Autodesk Inventor part; units mm, degrees
ref_plane "YZ Plane" through (0, 0, 0) normal (1, 0, 0) x (0, 1, 0)
ref_plane "XZ Plane" through (0, 0, 0) normal (0, 1, 0) x (-1, 0, 0)
ref_plane "XY Plane" through (0, 0, 0) normal (0, 0, 1) x (1, 0, 0)
sketch "Sketch1" plane through (0, 0, 0) normal (0, 1, 0) x (-1, 0, 0)
  line L0 (10, 67.88) -> (-10, 67.88)
  line L1 (-10, 67.88) -> (-10, -10)
  line L2 (-10, -10) -> (10, -10)
  line L3 (10, -10) -> (10, 67.88)
  point P0 (0, 0)
  dimension "d0" = 20
  dimension "d1" = 77.88
extrude "Extrusion1" add sketch "Sketch1" along normal blind 2
sketch "Sketch2" plane through (0, 2, 0) normal (0, 1, 0) x (1, 0, 0)
  line L0 (-10, -67.88) -> (10, -67.88)
  line L1 (0, -67.88) -> (-6.35, -67.88)
  line L2 (-6.35, -56.98) -> (6.35, -56.98)
  line L3 (6.35, -67.88) -> (0, -67.88)
  line L4 (10, 10) -> (-10, 10)
  line L5 (-6.35, -0.9) -> (6.35, -0.9)
  line L6 (-6.35, 10) -> (6.35, 10)
  line L7 (-6.35, -67.88) -> (-10, -67.88)
  line L8 (-10, 10) -> (-10, -67.88)
  line L9 (-10, -56.98) -> (-6.35, -56.98)
  line L10 (6.35, -67.88) -> (10, -67.88)
  line L11 (10, -67.88) -> (10, 10)
  line L12 (10, -56.98) -> (6.35, -56.98)
  line L13 (6.35, -0.9) -> (10, -0.9)
  line L14 (10, 10) -> (6.35, 10)
  line L15 (10, -0.9) -> (10, 10)
  line L16 (10, -67.88) -> (10, -56.98)
  line L17 (-10, -67.88) -> (-10, -56.98)
  line L18 (-6.35, -0.9) -> (-10, -0.9)
  line L19 (-10, -0.9) -> (-10, 10)
  line L20 (-10, 10) -> (-6.35, 10)
  point P0 (0, 0)
  dimension "d4" = 6.35
  dimension "d5" = 10.9
  dimension "d6" = 12.7
  dimension "d7" = 10.9
extrude "Extrusion2" add sketch "Sketch2" along normal blind 43.3354 contours L8 L9 L2 L12 L11 L0 | L8 L4 L11 L13 L5 L18
sketch "Sketch9" plane through (-10, 0, 67.88) normal (0, 0, 1) x (1, 0, 0)
  arc A0 (15.084, 37.3223) -> (4.684, 37.3223) centre (9.884, 37.3223) ccw
  line L0 (15.084, 30.9243) -> (15.084, 37.3223)
  line L1 (4.684, 36.1247) -> (4.684, 37.3223)
  arc A1 (15.084, 37.3223) -> (4.684, 37.3223) centre (9.884, 37.3223) ccw
  line L2 (4.684, 37.3223) -> (4.684, 30.9247)
  line L3 (9.8815, 15.3222) -> (-0.0013, 15.3222)
  line L4 (-0.0013, 25.726) -> (-0.0013, 15.3222)
  line L5 (4.684, 30.9247) -> (4.684, 25.726)
  line L6 (15.084, 30.9243) -> (15.0845, 20.5254)
  arc A2 (15.084, 30.9243) -> (15.084, 30.9251) centre (9.884, 30.9244) ccw
  line L7 (4.684, 25.726) -> (-0.0013, 25.726)
  arc A3 (9.8815, 15.3222) -> (15.0845, 20.5254) centre (9.8815, 20.5252) ccw
  line L8 (0, 0) -> (20, 0)
  line L9 (0, 45.3354) -> (20, 45.3354)
  point P0 (10, 0)
  point P1 (2.3413, 25.726)
  point P2 (15.084, 30.9247)
  point P3 (9.884, 42.5223)
  point P4 (-0.0013, 20.5241)
  point P5 (10, 45.3354)
  dimension "d76" = 15.3222
  dimension "d77" = 10.4039
  dimension "d78" = 10.4
  dimension "d79" = 27.2001
  dimension "d80" = 15.0858
  dimension "d81" = 8.0131
fillet "Fillet4" radius 10 4 edges at (10, 45.3354, 62.43) (-10, 45.3354, 62.43) (-10, 45.3354, -4.55) (10, 45.3354, -4.55)
sketch "Sketch10" plane through (0, 2, 0) normal (0, 1, 0) x (1, 0, 0)
  line L0 (10, -67.88) -> (-10, -67.88)
  line L1 (-10, 10) -> (10, 10)
  line L2 (10, -56.98) -> (10, -0.9)
  line L3 (-10, -0.9) -> (-10, -56.98)
  line L4 (10, -28.94) -> (-10, -28.94)
  circle A0 centre (0, -28.94) radius 2.125
  point P0 (0, 0)
  dimension "d53" = 77.88
  dimension "d54" = 4.25
extrude "Extrusion10" cut sketch "Sketch10" against normal blind 2
extrude "Extrusion11" cut sketch "Sketch9" against normal through all
sketch "Sketch11" plane through (10, 0, 67.88) normal (1, 0, 0) x (0, 0, -1)
  line L0 (0, 0) -> (0, 15.3222)
  line L1 (77.88, 25.726) -> (77.88, 35.3354)
  line L2 (0, 0) -> (77.88, 0)
  line L3 (77.88, 0) -> (77.88, 35.3354)
  line L4 (77.88, 35.3354) -> (0, 35.3354)
  line L5 (0, 35.3354) -> (0, 0)
  point P0 (67.88, 0)
extrude "Extrusion12" add sketch "Sketch11" along normal blind 2
sketch "Sketch12" plane through (12, 0, 67.88) normal (1, 0, 0) x (0, 0, -1)
  line L0 (10.9, 35.3354) -> (0, 35.3354)
  line L1 (77.88, 25.726) -> (77.88, 35.3354)
  line L2 (0, 35.3354) -> (77.88, 35.3354)
  line L3 (77.88, 35.3354) -> (0, 35.3354)
  line L4 (38.94, 35.3354) -> (64.34, 35.3354)
  line L5 (38.94, 35.3354) -> (13.54, 35.3354)
  line L6 (77.88, 0) -> (0, 0)
  line L7 (13.54, 35.3354) -> (64.34, 35.3354)
  line L8 (64.34, 35.3354) -> (64.34, 0)
  line L9 (64.34, 0) -> (13.54, 0)
  line L10 (13.54, 0) -> (13.54, 35.3354)
  line L11 (13.54, 0) -> (31.84, 0)
  line L12 (31.84, 0) -> (31.84, 6)
  arc A0 (33.34, 31.3354) -> (30.34, 31.3354) centre (31.84, 31.3354) ccw
  arc A1 (30.34, 6) -> (33.34, 6) centre (31.84, 6) ccw
  line L13 (30.34, 31.3354) -> (30.34, 6)
  line L14 (33.34, 31.3354) -> (33.34, 6)
  line L15 (31.84, 31.3354) -> (13.54, 31.3354)
  point P0 (67.88, 0)
  dimension "d65" = 25.4
  dimension "d66" = 25.4
  dimension "d67" = 50.8
  dimension "d68" = 18.3
  dimension "d69" = 6
  dimension "d71" = 3
  dimension "d72" = 3
  dimension "d75" = 18.3
extrude "Extrusion13" cut sketch "Sketch12" against normal blind 2 contours A0 L14 A1 L13
properties part number "6 Backet Adjustment 3.0"
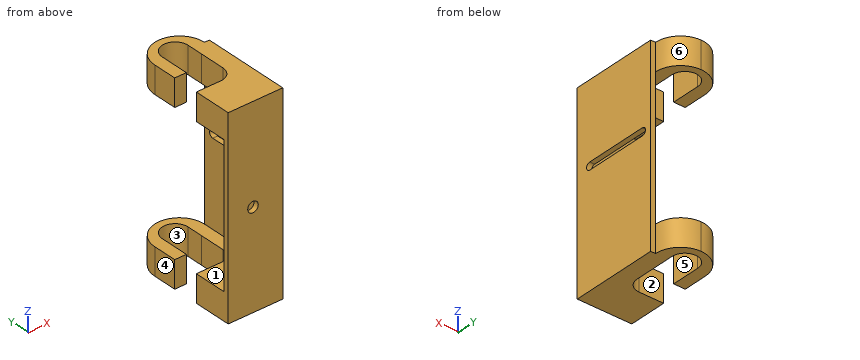
Design review of the part built by this model. Coordinates are the model's own, in mm. Face numbers are marked on the shaded views. A direction names the side the tool comes from. Round coordinates to 2 decimals unless told otherwise and drop trailing zeros. Write each loop counter-clockwise with the first axis right and the second up, starting at its lowest first coordinate (ties: lowest second). Pieces come first, ordered by that corner, then holes. Notation, with made-up numbers: (24.25, 33) -> (75.25, 33) arc R26 cw to (75.25, 72) -> close; hole circle Ø9 at (23, 85). An arc over 180 degrees is marked (long way). Answer in a Markdown table with one row per item.
Q1. For the marked faces 1, 2 and 3, list the 3-axis set-ups (+Z, -Z, +X, -X, +Y, -Y) from which the entire face can be reached by the end or side of a thin tool; tool diameter is ignored.
The answers:
| item | result |
|---|---|
| face 1 | -X, +Y |
| face 2 | +Z, -Z, -X |
| face 3 | +Z, -Z |
Q2. Clearance check with flat-ended pins moving along their axes: pin 1 Ø10 at (x, z) = (3.5, 27.5) entering from +Y; pin 2 Ø8 at (x, y) = (0, 37.5) entering from +Z; pin 3 Ø5 at (x, z) = (-6, -2.5) entering from +Y; pin 4 Ø1 at (x, z) = (11.5, 13) entering from +Y. State where each tip first meets the part, or that it passes through.
The answers:
| item | result |
|---|---|
| pin 1 | y = 2 |
| pin 2 | through |
| pin 3 | y = 44.7 |
| pin 4 | y = 35.34 |
Q3. To check wall thickness, follow L1, parallel to Z at x = 0, y = 1.05 (3 decimals); L2, parallel to Z at x = 5, y = 5.5; L3, parallel to Y at x = 10.5, z = 36. State the ranges of each line that lie inside material, in increasing order. Write a range as [from, to].
The answers:
| item | result |
|---|---|
| L1 | [-10, 26.815], [31.065, 67.88] |
| L2 | [-10, 0.9], [56.98, 67.88] |
| L3 | [0, 4.5], [32.83, 35.34] |
Q4. Take a section at A-A, the plane z = 28.94. State the section outline as (x, y) points (1 decimal).
The answers:
| item | result |
|---|---|
| outline | (-10, 0) -> (-2.1, 0) -> (-2.1, 2) -> (-10, 2) -> close; (2.1, 0) -> (12, 0) -> (12, 35.3) -> (10, 35.3) -> (10, 2) -> (2.1, 2) -> close |
Q5. Take a section at B-B, the plane y = 9. State the section outline as (x, z) points, then the cut area to 3 significant figures.
The answers:
| item | result |
|---|---|
| outline | (-10, -10) -> (12, -10) -> (12, 34.54) -> (10, 34.54) -> (10, 0.9) -> (-10, 0.9) -> close; (-10, 56.98) -> (10, 56.98) -> (10, 37.54) -> (12, 37.54) -> (12, 67.88) -> (-10, 67.88) -> close |
| area | 586 mm² |
Q6. Take a section at D-D, the plane y = 28.5. State the section outline as (x, z) points.
The answers:
| item | result |
|---|---|
| outline | (-10, -10) -> (-5.32, -10) -> (-5.32, 0.9) -> (-10, 0.9) -> close; (-10, 56.98) -> (-5.32, 56.98) -> (-5.32, 67.88) -> (-10, 67.88) -> close; (5.08, -10) -> (12, -10) -> (12, 34.54) -> (10, 34.54) -> (10, 0.9) -> (5.08, 0.9) -> close; (5.08, 56.98) -> (10, 56.98) -> (10, 37.54) -> (12, 37.54) -> (12, 67.88) -> (5.08, 67.88) -> close |
Q7. Take a section at C-C, the plane x = 3.75. State the section outline as (y, z) points.
The answers:
| item | result |
|---|---|
| outline | (0, -10) -> (17.05, -10) -> (17.05, 0.9) -> (2, 0.9) -> (2, 56.98) -> (17.05, 56.98) -> (17.05, 67.88) -> (0, 67.88) -> close; (40.8, -10) -> (44.61, -10) -> (44.61, 0.9) -> (40.8, 0.9) -> close; (40.8, 56.98) -> (44.61, 56.98) -> (44.61, 67.88) -> (40.8, 67.88) -> close |
Q8. Draft analysis for pull direction Y (two halves, no side actions). For the marked faces 4, 5 and 6, state which applies: +Y half, -Y half, draft (parallel to the pull), parting line (faces both ways), or undercut.
The answers:
| item | result |
|---|---|
| face 4 | draft |
| face 5 | undercut |
| face 6 | +Y half |
